Source: CAD feature listing. Evaluate the final solid. Frame: model axes, mm. Give positions to 0.01 mm unless a question says otherwise; leave off trailing zeros. Loops run counter-clockwise (first coordinate to the right, second up) from the corner with the lowest first, then second, coordinate; pieces in that order, holes last. Notation, with made-up numbers: M 23.5,5 L 52.5,5 A31 cw 52.5,37 Z; hole C 77,37 d2. An arc over 180 degrees is marked long. Write item = value, one per line.
from build123d import *
from OCP.BRepFilletAPI import BRepFilletAPI_MakeFillet

# Parameters (mm, degrees)
CUT_EXTRUDE1_START         = -1.5
CUT_EXTRUDE1_DEPTH         = 1.5
CUT_EXTRUDE2_DEPTH         = 56.320855182
CUT_EXTRUDE3_DEPTH         = 56.320855182
FILLET1_R1                 = 2
FILLET1_R2                 = 1.5
FILLET1_R3                 = 1.5
FILLET1_R4                 = 1.5
FILLET1_R5                 = 1
FILLET1_R6                 = 1
FILLET1_R7                 = 0.3
F_2_0_2_DIAMETER_HOLE1_D   = 2
F_2_5_2_5_DIAMETER_HOLE1_D = 2.5
F_3_2_3_2_DIAMETER_HOLE1_D = 3.2


with BuildPart() as part:
    # Cut-Extrude1: read off the stored shape, not the designer's step
    # Cut-Extrude1 outline → Cut-Extrude1 (new body)
    with BuildSketch(Plane.XY.offset(1.5).offset(CUT_EXTRUDE1_START)):
        with BuildLine():
            Line((-21.15922941, 42.990956489), (-21.918524362, 42.593852668))
            Line((-21.918524362, 42.593852668), (-22.331690837, 37.008180338))
            Line((-22.331690837, 37.008180338), (-15.823880633, 32.753073704))
            Line((-15.823880633, 32.753073704), (-14.767696121, 28.083626208))
            Line((-14.767696121, 28.083626208), (-16.26955663, 25.9101387))
            Line((-16.26955663, 25.9101387), (-13.325866142, 14.548277254))
            Line((-13.325866142, 14.548277254), (-11.044500218, 13.256714261))
            Line((-11.044500218, 13.256714261), (-9.843169723, 8.619898436))
            Line((-9.843169723, 8.619898436), (-18.106030722, -5.122739041))
            Line((-18.106030722, -5.122739041), (-17.064214449, -9.58485809))
            Line((-17.064214449, -9.58485809), (-12.690100502, -12.329039203))
            Line((-12.690100502, -12.329039203), (-8.962822896, -11.10580142))
            Line((-8.962822896, -11.10580142), (-7.911354227, -9.756154848))
            Line((-7.911354227, -9.756154848), (-1.053266461, -8.076943446))
            Line((-1.053266461, -8.076943446), (0.097779189, -8.690341842))
            Line((0.097779189, -8.690341842), (3.254584825, -8.251896615))
            Line((3.254584825, -8.251896615), (5.068180176, -7.125558451))
            Line((5.068180176, -7.125558451), (6.906602667, -3.594529202))
            Line((6.906602667, -3.594529202), (5.391678643, 2.702231034))
            Line((5.391678643, 2.702231034), (8.443636754, 11.032011447))
            Line((8.443636754, 11.032011447), (6.916630149, 13.34590119))
            Line((6.916630149, 13.34590119), (13.586412116, 31.791123225))
            Line((13.586412116, 31.791123225), (16.484018961, 32.532910561))
            Line((16.484018961, 32.532910561), (19.81145552, 41.346140579))
            Line((19.81145552, 41.346140579), (15.452897729, 50.590933994))
            Line((15.452897729, 50.590933994), (8.66072149, 50.590933994))
            Line((8.66072149, 50.590933994), (8.66072149, 44.490933994))
            Line((8.66072149, 44.490933994), (9.66072149, 44.490933994))
            ThreePointArc((9.66072149, 44.490933994), (10.615066101, 43.192226171), (9.090581088, 42.66938672))
            Line((9.090581088, 42.66938672), (8.890254379, 39.021331889))
            Line((8.890254379, 39.021331889), (3.686776041, 39.121354833))
            Line((3.686776041, 39.121354833), (2.58727318, 42.990956489))
            Line((2.58727318, 42.990956489), (-21.15922941, 42.990956489))
        make_face()
        with BuildLine():
            ThreePointArc((-3.894243345, -3.831676855), (-5.608872185, -2.248942531), (-4.026137862, -0.534313691))
            Line((-4.026137862, -0.534313691), (-0.677019452, -0.400348965))
            ThreePointArc((-0.677019452, -0.400348965), (1.037609388, -1.983083289), (-0.545124935, -3.697712129))
            Line((-0.545124935, -3.697712129), (-3.894243345, -3.831676855))
        make_face(mode=Mode.SUBTRACT)
    extrude(amount=CUT_EXTRUDE1_DEPTH)

    # Sketch2 → Cut-Extrude2 (cut, through all)
    with BuildSketch(Plane.XY.offset(1.5)):
        with BuildLine():
            Line((-8.400629557, -3.479539033), (-12.328216542, -2.729986131))
            ThreePointArc((-12.328216542, -2.729986131), (-14.258274586, -4.041426541), (-12.946834177, -5.971484585))
            Line((-12.946834177, -5.971484585), (-9.019247192, -6.721037486))
            ThreePointArc((-9.019247192, -6.721037486), (-7.089189148, -5.409597077), (-8.400629557, -3.479539033))
        make_face()
    extrude(amount=-CUT_EXTRUDE2_DEPTH, mode=Mode.SUBTRACT)

    # Sketch3 → Cut-Extrude3 (cut, through all)
    with BuildSketch(Plane(origin=(0, 0, 0), x_dir=(-1, 0, 0), z_dir=(0, 0, -1))):
        Polygon((-1.669040668, 13.788566276), (0.421242883, 7.902808428), (2.674335505, 7.270595549), (4.846116127, 8.142081874), (6.289526399, 14.218922957), (5.51540188, 15.234387716), (6.801285994, 20.3627961), (7.865027392, 20.96090236), (8.717011471, 24.560534964), (5.714933344, 28.35768306), (-2.622436807, 27.906842737), (-5.197547994, 23.808110114), (-3.962369217, 20.321340098), (-2.840334409, 19.841428909), (-1.008931735, 14.881586698), align=None)
    extrude(amount=-CUT_EXTRUDE3_DEPTH, mode=Mode.SUBTRACT)

    # Fillet1: one fillet with a radius per group of edges: ONE call of the kernel's fillet builder (fillet() takes one radius for all edges)
    fillet1_edges_1 = [part.edges().sort_by_distance(p)[0] for p in [
        (8.66072149, 50.590933994, 0.75),
    ]]
    fillet1_edges_2 = [part.edges().sort_by_distance(p)[0] for p in [
        (-13.325866142, 14.548277254, 0.75),
        (2.58727318, 42.990956489, 0.75),
        (8.890254379, 39.021331889, 0.75),
        (-8.962822896, -11.10580142, 0.75),
        (-17.064214449, -9.58485809, 0.75),
        (-9.843169723, 8.619898436, 0.75),
        (-15.823880633, 32.753073704, 0.75),
        (13.586412116, 31.791123225, 0.75),
        (-12.690100502, -12.329039203, 0.75),
        (8.443636754, 11.032011447, 0.75),
        (-18.106030722, -5.122739041, 0.75),
        (5.391678643, 2.702231034, 0.75),
        (-11.044500218, 13.256714261, 0.75),
        (6.906602667, -3.594529202, 0.75),
        (-16.26955663, 25.9101387, 0.75),
        (3.686776041, 39.121354833, 0.75),
        (3.254584825, -8.251896615, 0.75),
        (16.484018961, 32.532910561, 0.75),
        (0.097779189, -8.690341842, 0.75),
        (-7.911354227, -9.756154848, 0.75),
        (-14.767696121, 28.083626208, 0.75),
    ]]
    fillet1_edges_3 = [part.edges().sort_by_distance(p)[0] for p in [
        (15.452897729, 50.590933994, 0.75),
        (19.81145552, 41.346140579, 0.75),
    ]]
    fillet1_edges_4 = [part.edges().sort_by_distance(p)[0] for p in [
        (-1.053266461, -8.076943446, 0.75),
        (6.916630149, 13.34590119, 0.75),
        (5.068180176, -7.125558451, 0.75),
    ]]
    fillet1_edges_5 = [part.edges().sort_by_distance(p)[0] for p in [
        (-6.801285994, 20.3627961, 0.75),
        (5.197547994, 23.808110114, 0.75),
    ]]
    fillet1_edges_6 = [part.edges().sort_by_distance(p)[0] for p in [
        (1.008931735, 14.881586698, 0.75),
        (1.669040668, 13.788566276, 0.75),
        (-21.918524362, 42.593852668, 0.75),
        (2.840334409, 19.841428909, 0.75),
        (-22.331690837, 37.008180338, 0.75),
        (-0.421242883, 7.902808428, 0.75),
        (-6.289526399, 14.218922957, 0.75),
        (-2.674335505, 7.270595549, 0.75),
        (-5.51540188, 15.234387716, 0.75),
        (-4.846116127, 8.142081874, 0.75),
        (3.962369217, 20.321340098, 0.75),
        (2.622436807, 27.906842737, 0.75),
        (-7.865027392, 20.96090236, 0.75),
        (-5.714933344, 28.35768306, 0.75),
        (-8.717011471, 24.560534964, 0.75),
    ]]
    fillet1_edges_7 = [part.edges().sort_by_distance(p)[0] for p in [
        (9.090581088, 42.66938672, 0.75),
    ]]
    fillet1 = BRepFilletAPI_MakeFillet(part.part.solid().wrapped)
    for e in fillet1_edges_1:
        fillet1.Add(FILLET1_R1, e.wrapped)
    for e in fillet1_edges_2:
        fillet1.Add(FILLET1_R2, e.wrapped)
    for e in fillet1_edges_3:
        fillet1.Add(FILLET1_R3, e.wrapped)
    for e in fillet1_edges_4:
        fillet1.Add(FILLET1_R4, e.wrapped)
    for e in fillet1_edges_5:
        fillet1.Add(FILLET1_R5, e.wrapped)
    for e in fillet1_edges_6:
        fillet1.Add(FILLET1_R6, e.wrapped)
    for e in fillet1_edges_7:
        fillet1.Add(FILLET1_R7, e.wrapped)
    add(Compound.cast(fillet1.Shape()), mode=Mode.REPLACE)

    # Ø2.0 (2) Diameter Hole1 (through all)
    with Locations(Plane(origin=(0, 0, 0), x_dir=(-1, 0, 0), z_dir=(0, 0, -1))):
        with Locations((19.749063689, 41.009673781)):
            Hole(F_2_0_2_DIAMETER_HOLE1_D / 2)

    # Ø2.5 (2.5) Diameter Hole1 (through all)
    with Locations(Plane(origin=(0, 0, 0), x_dir=(-1, 0, 0), z_dir=(0, 0, -1))):
        with Locations((-13.25072149, 47.590933994)):
            Hole(F_2_5_2_5_DIAMETER_HOLE1_D / 2)

    # Ø3.2 (3.2) Diameter Hole1 (through all)
    with Locations(Plane(origin=(0, 0, 0), x_dir=(-1, 0, 0), z_dir=(0, 0, -1))):
        with Locations((3.676270681, 32.308049922)):
            Hole(F_3_2_3_2_DIAMETER_HOLE1_D / 2)


solid = part.part
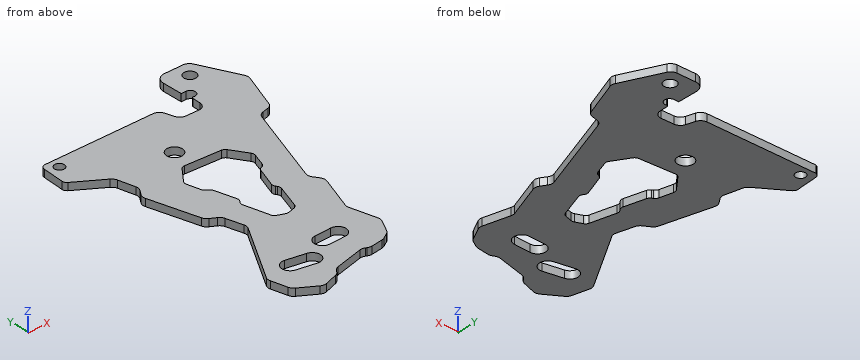
1. First-contact query: pin 1 Ø0.8 at (y, z) = (46, 1) entering from -X; pin 2 Ø1.2 at (x, y) = (9.66, 43.49) entering from -Z. Flat tips, straight axial feed; report the tip coordinate or a pass-through.
Derived:
pin_1 = 8.66
pin_2 = through
2. Cut plane A-A, the plane y = 17.5. Return the cut outline in (x, z).
Derived:
outline = M -14.09,0 L -6.08,0 L -6.08,1.5 L -14.09,1.5 Z; M 1.98,0 L 8.42,0 L 8.42,1.5 L 1.98,1.5 Z
3. Cut plane B-B, the plane z = 1.15. Count the separate pieces of the cut face and the enclosed holes in it, then the cut area to 3 significant figures.
Derived:
separate_pieces = 1
enclosed_holes = 6
area = 1,160 mm²
4. Material intervals for probe 1 along Y at (x, z) = (-1, 0.7); probe 2 along Y at (x, z) = (-12.5, 1.05); probe 3 along Y at (x, z) = (-16.5, 0.9), sorted ascending. Write a range as from..to.
Derived:
probe_1 = -8.19..-3.72, -0.41..7.74, 28.1..42.99
probe_2 = -12.18..-6.06, -2.71..4.2, 14.08..42.99
probe_3 = -9.94..-2.45, 33.2..42.99
